The model under review builds one solid part; all positions refer to its coordinate system, in mm. A direction names the side the tool comes from. Give positions to 0.01 mm unless a question says otherwise; leave off trailing zeros. Order: outer loops, then holes, each group sorted by start corner. A loop starts at its lowest first (then second) coordinate and runs counter-clockwise, first axis right, second up.
```python
from build123d import *

# Parameters (mm, degrees)
F1_DEPTH = 41.5
F2_DEPTH = 40.5
F3_DEPTH = 3
F4_DEPTH = 0.1
F5_DEPTH = 3.5
F6_R     = 5
F7_R     = 3


with BuildPart() as f1:
    # F0 (on Right) → F1 (new body)
    with BuildSketch(Plane.YZ):
        Polygon((0, 9), (0, 0), (6.5, 0), (6.5, 3), (10, 3), (10, 5.8), (6.5, 5.8), (6.5, 9), align=None)
    extrude(amount=F1_DEPTH)

    # F2 (add): a face of the model
    f2_faces = [f1.faces().sort_by_distance(p)[0] for p in [
        (0, 3.9674231332, 4.4856515373),
    ]]
    extrude(f2_faces, amount=F2_DEPTH)

    # F3 (add): a face of the model
    f3_faces = [f1.faces().sort_by_distance(p)[0] for p in [
        (0.5, 3.25, 0),
    ]]
    extrude(f3_faces, amount=F3_DEPTH)

    # F4 (add): a face of the model
    f4_faces = [f1.faces().sort_by_distance(p)[0] for p in [
        (0.5, 8.25, 5.8),
    ]]
    extrude(f4_faces, amount=F4_DEPTH)

    # F5 (add): a face of the model
    f5_faces = [f1.faces().sort_by_distance(p)[0] for p in [
        (0.5, 0, 3),
    ]]
    extrude(f5_faces, amount=F5_DEPTH)

    # F6
    f6_edges = [f1.edges().sort_by_distance(p)[0] for p in [
        (41.5, -3.5, 3),
        (-40.5, -3.5, 3),
    ]]
    fillet(f6_edges, radius=F6_R)

    # F7
    f7_edges = [f1.edges().sort_by_distance(p)[0] for p in [
        (0.5, -3.5, 9),
        (0.5, -3.5, -3),
    ]]
    fillet(f7_edges, radius=F7_R)


solid = f1.part
```
1. For faces 1 (the flat face through (1, 8, 5.9)), 2 (the cylindrical face through (1, -2.6, -2.14)), 3 (the flat face through (1, 8, 3)), list the 3-axis set-ups (+Z, -Z, +X, -X, +Y, -Y) from which the entire face can be reached by the end or side of a thin tool; tool diameter is ignored.
2. Take a section at B-B (z = 1.5). Write out the cut boundary in (x, y).
3. Insertion check: pin 1 (1 mm diameter, centred on x = -12, y = 8, fed in from +Z); pin 2 (1.8 mm diameter, centred on x = 19, y = 8.5, fed in from -Z); pin 3 (3 mm diameter, centred on x = -14.5, z = 1, fed in from +Y). Each pin has a flat end and moves straight along its axis. Give the tip position at first contact, or say it passes through.
4. Take a section at A-A (x = -16). Write out the cut boundary in (y, z), and give its area (3 significant figures).
5. To check wall thickness, follow line 1 (Y direction, x = 15.5, z = 1.5); line 2 (Z direction, x = 33.5, y = 8.75); line 3 (X direction, y = -1.25, z = 6.5). State the ranges of each line that lie inside material, in increasing order.
6. Take a section at C-C (y = 8.5). Write out the cut boundary in (x, z), and give its area (3 significant figures).
Answer:
1. face 1: +Z, +X, -X, +Y
1. face 2: -Z, +X, -X, -Y
1. face 3: -Z, +X, -X, +Y
2. outline: (-40.5, 1.5) arc R5 ccw to (-35.5, -3.5) - (36.5, -3.5) arc R5 ccw to (41.5, 1.5) - (41.5, 6.5) - (-40.5, 6.5) - close
3. pin 1: stops at z = 5.9
3. pin 2: stops at z = 3
3. pin 3: stops at y = 6.5
4. outline: (-3.5, 0) arc R3 ccw to (-0.5, -3) - (6.5, -3) - (6.5, 3) - (10, 3) - (10, 5.9) - (6.5, 5.9) - (6.5, 9) - (-0.5, 9) arc R3 ccw to (-3.5, 6) - close
4. area: 126 mm2
5. line 1: y = -3.5 to 6.5
5. line 2: z = 3 to 5.9
5. line 3: x = -39.63 to 40.63
6. outline: (-40.5, 3) - (41.5, 3) - (41.5, 5.9) - (-40.5, 5.9) - close
6. area: 238 mm2
